Can you work these out from the model? Positions are in its coordinate system, mm. A direction names the side the tool comes from. Round coordinates to 2 decimals unless told otherwise and drop trailing zeros. Loops run counter-clockwise (first coordinate to the right, second up) from the corner with the lowest first, then second, coordinate; pieces in that order, holes last. Notation, with made-up numbers: M -11.75,73.5 L 33.25,73.5 A11 ccw 33.25,86.5 Z; hole C -21,60 d1. An arc over 180 degrees is marked long. Return JSON: item names as keys, results as strings.
Autodesk Inventor part; units mm, degrees
ref_plane "YZ Plane" through (0, 0, 0) normal (1, 0, 0) x (0, 1, 0)
ref_plane "XZ Plane" through (0, 0, 0) normal (0, 1, 0) x (-1, 0, 0)
ref_plane "XY Plane" through (0, 0, 0) normal (0, 0, 1) x (1, 0, 0)
sketch "Sketch1" plane through (0, 0, 0) normal (0, 0, 1) x (1, 0, 0)
  arc A0 (-16, 0) -> (-12, -4) centre (-12, 0) ccw
  arc A1 (-8, 8) -> (-16, 8) centre (-12, 8) ccw
  line L0 (-16, 0) -> (-16, 8)
  line L1 (-8, 8) -> (-8, 4)
  arc A2 (12, -4) -> (12, 4) centre (12, 0) ccw
  line L2 (-12, -4) -> (12, -4)
  line L3 (12, 4) -> (-8, 4)
  line L4 (-23.3941, 0) -> (22.5657, 0)
  line L5 (0, -8.1941) -> (0, 15.3657)
  point P0 (0, 0)
  dimension "d3" = 4
  dimension "d4" = 4
  dimension "d5" = 4
  dimension "d6" = 24
  dimension "d7" = 8
  dimension "d10" = 0
  dimension "d12" = 90
  dimension "d14" = 4
  dimension "d15" = 4
  dimension "d16" = 12
  dimension "d123" = 12
extrude "Extrusion1" add sketch "Sketch1" along normal blind 8
sketch "Sketch13" plane through (0, 0, 8) normal (0, 0, 1) x (1, 0, 0)
  arc A0 (12, -4) -> (12, 4) centre (12, 0) ccw
  line L0 (-8, 8) -> (-8, 4)
  arc A1 (9.1716, 1) -> (9.1716, -1) centre (12, 0) ccw
  arc A2 (11, -2.8284) -> (13, -2.8284) centre (12, 0) ccw
  arc A3 (14.8284, -1) -> (14.8284, 1) centre (12, 0) ccw
  arc A4 (13, 2.8284) -> (11, 2.8284) centre (12, 0) ccw
  line L1 (14.8284, 1) -> (13, 1)
  line L2 (11, 1) -> (9.1716, 1)
  line L3 (11, -2.8284) -> (11, -1)
  line L4 (11, 1) -> (11, 2.8284)
  line L5 (14.8284, -1) -> (13, -1)
  line L6 (11, -1) -> (9.1716, -1)
  line L7 (13, -2.8284) -> (13, -1)
  line L8 (13, 1) -> (13, 2.8284)
  point P0 (0, 0)
  dimension "d125" = 3
  dimension "d126" = 3
  dimension "d127" = 3
  dimension "d128" = 3
  dimension "d129" = 2
  dimension "d130" = 2
  dimension "d131" = 2
  dimension "d132" = 2
  dimension "d133" = 1
  dimension "d134" = 1
  dimension "d135" = 1
  dimension "d136" = 1
extrude "Extrusion13" cut sketch "Sketch13" against normal through all
sketch "Sketch14" plane through (0, 0, 8) normal (0, 0, 1) x (1, 0, 0)
  arc A0 (-16, 0) -> (-12, -4) centre (-12, 0) ccw
  line L0 (-8, 4) -> (12, 4)
  arc A1 (-8, 8) -> (-16, 8) centre (-12, 8) ccw
  circle A2 centre (-12, 0) radius 2.5
  circle A3 centre (-12, 8) radius 2.5
  circle A4 centre (-4, 0) radius 2.5
  circle A5 centre (4, 0) radius 2.5
  point P0 (0, 0)
  dimension "d139" = 5
  dimension "d140" = 5
  dimension "d146" = 8
extrude "Extrusion14" cut sketch "Sketch14" against normal through all
sketch "Sketch15" plane through (0, 0, 8) normal (0, 0, 1) x (1, 0, 0)
  circle A0 centre (4, 0) radius 2.5
  circle A1 centre (-4, 0) radius 2.5
  circle A2 centre (-12, 8) radius 2.5
  circle A3 centre (-12, 0) radius 2.5
  arc A4 (-16, 0) -> (-12, -4) centre (-12, 0) ccw
  arc A5 (-8, 8) -> (-16, 8) centre (-12, 8) ccw
  circle A6 centre (-12, 0) radius 3
  circle A7 centre (-4, 0) radius 3
  circle A8 centre (4, 0) radius 3
  circle A9 centre (-12, 8) radius 3
  point P0 (0, 0)
  dimension "d150" = 6
  dimension "d151" = 6
  dimension "d152" = 6
  dimension "d153" = 6
extrude "Extrusion15" cut sketch "Sketch15" against normal blind 0.8
sketch "Sketch16" plane through (0, 0, 0) normal (0, 0, -1) x (-1, 0, 0)
  circle A0 centre (-4, 0) radius 2.5
  circle A1 centre (4, 0) radius 2.5
  circle A2 centre (12, 8) radius 2.5
  circle A3 centre (12, 0) radius 2.5
  arc A4 (12, -4) -> (16, 0) centre (12, 0) ccw
  arc A5 (16, 8) -> (8, 8) centre (12, 8) ccw
  circle A6 centre (12, 8) radius 3
  circle A7 centre (12, 0) radius 3
  circle A8 centre (4, 0) radius 3
  circle A9 centre (-4, 0) radius 3
  point P0 (0, 0)
  dimension "d156" = 6
  dimension "d157" = 6
  dimension "d158" = 6
  dimension "d159" = 6
extrude "Extrusion16" cut sketch "Sketch16" against normal blind 0.8
sketch "Sketch17" plane through (0, 0, 8) normal (0, 0, 1) x (1, 0, 0)
  circle A0 centre (-12, 8) radius 3
  circle A1 centre (-4, 0) radius 3
  circle A2 centre (-12, 0) radius 3
  arc A3 (-16, 0) -> (-12, -4) centre (-12, 0) ccw
  line L0 (-8, 4) -> (12, 4)
  line L1 (-8, 8) -> (-8, 4)
  arc A4 (-8, 8) -> (-16, 8) centre (-12, 8) ccw
  arc A5 (-10.1972, -3) -> (-10.1972, 3) centre (-12, 0) ccw
  arc A6 (-5.8028, 3) -> (-5.8028, -3) centre (-4, 0) ccw
  arc A7 (-15, 6.1972) -> (-9, 6.1972) centre (-12, 8) ccw
  line L2 (-10.1972, 3) -> (-5.8028, 3)
  line L3 (-10.1972, -3) -> (-5.8028, -3)
  line L4 (-15, 6.1972) -> (-15, 4)
  line L5 (-9, 6.1972) -> (-9, 4)
  line L6 (-15, 4) -> (-9, 4)
  arc A8 (-2.1972, -3) -> (-2.1972, 3) centre (-4, 0) ccw
  arc A9 (2.1972, 3) -> (2.1972, -3) centre (4, 0) ccw
  line L7 (-2.1972, 3) -> (2.1972, 3)
  line L8 (-2.1972, -3) -> (2.1972, -3)
  arc A10 (5.8028, -3) -> (5.8028, 3) centre (4, 0) ccw
  arc A11 (10.1972, 3) -> (10.1972, -3) centre (12, 0) ccw
  line L9 (5.8028, 3) -> (10.1972, 3)
  line L10 (5.8028, -3) -> (10.1972, -3)
  point P0 (0, 0)
  dimension "d162" = 7
  dimension "d163" = 7
  dimension "d164" = 7
  dimension "d165" = 6
  dimension "d166" = 4
  dimension "d172" = 8
extrude "Extrusion17" cut sketch "Sketch17" against normal through all contours A5 L2 A6 L3 | A7 L5 L6 L4 | A8 L7 A9 L8 | A10 L9 A11 L10
properties part number "5MRA Beam"
Q1. Suppose I cut it at A-A, the plane x = 4. Please give me the cut outline in (y, z).
Results:
{"outline": "M -4,0 L -3,0 L -3,0.8 L -2.5,0.8 L -2.5,7.2 L -3,7.2 L -3,8 L -4,8 Z; M 2.5,0.8 L 3,0.8 L 3,0 L 4,0 L 4,8 L 3,8 L 3,7.2 L 2.5,7.2 Z"}
Q2. On a 3-axis mill with a long thin cutter (end or side, diameter ignored), from which of +Z, -Z, +X, -X, +Y, -Y can I reach the whole of each face in a straight line? I mean faces 1 (the flat face through (-10, 10, 0.8)), 2 (the flat face through (10, 1, 4)), 3 (the cylindrical face through (-14.4, -1.8, 7.6)). Say none if no direction works.
Results:
{"face 1": "-Z", "face 2": "+Z, -Z", "face 3": "+Z"}
Q3. I'm going to push flat-ended pins straight in: pin 1 Ø4 at (x, z) = (9, 3.5) entering from +Y; pin 2 Ø1.8 at (x, y) = (5, 0.5) entering from -Z; pin 3 Ø3 at (y, z) = (7.5, 4) entering from +X; pin 4 Ø2 at (y, z) = (-2, 5) entering from +X. Where does each tip first touch, or does it pass through?
Results:
{"pin 1": "stops at y = 4", "pin 2": "passes through", "pin 3": "stops at x = -8", "pin 4": "stops at x = 15.87"}
Q4. Suppose I cut it at D-D, the plane x = -5. Please give me the cut outline in (y, z).
Results:
{"outline": "M -4,0 L -2.83,0 L -2.83,0.8 L -2.29,0.8 L -2.29,7.2 L -2.83,7.2 L -2.83,8 L -4,8 Z; M 2.29,0.8 L 2.83,0.8 L 2.83,0 L 4,0 L 4,8 L 2.83,8 L 2.83,7.2 L 2.29,7.2 Z"}
Q5. Suppose I cut it at B-B, the plane z = 5. State how many separate pieces and enclosed holes the cut face has, plus the area to 3 significant figures.
Results:
{"separate pieces": "1", "enclosed holes": "9", "area": "163 mm2"}
Q6. If I drill on line 1 along Y through (x, z) = (-12, 0.6); line 2 along Y through (x, z) = (-4, 3.25); line 3 along Y through (x, z) = (-4, 7.4), over which ranges is the centre line in solid material (lowest first)?
Results:
{"line 1": "y = -4 to -3, 3 to 4, 4.5 to 5, 11 to 12", "line 2": "y = -4 to -2.5, 2.5 to 4", "line 3": "y = -4 to -3, 3 to 4"}
Q7. Thinking about a two-plate mould opening in Z: for faces 4 (the flat face through (-2, 2, 0.8)), 5 (the cylindrical face through (9, 0, 4)), 6 (the flat face through (-14, 2, 7.2)), which applies, pulls with the +Z half, pulls with the -Z half, needs draft (parallel to the pull), parting line crosses it, or undercut?
Results:
{"face 4": "pulls with the -Z half", "face 5": "needs draft", "face 6": "pulls with the +Z half"}
